from build123d import *

# Parameters (mm, degrees)
SKETCH_W        = 13.8
SKETCH_H        = 7.2
SKETCH_R        = 2.6
SKETCH_R_2      = 1.7
PAD_DEPTH       = 3
SKETCH001_R     = 2.6
SKETCH001_R_2   = 1.7
PAD001_DEPTH    = 20
CHAMFER_SIZE    = 0.5
CHAMFER001_SIZE = 0.5
CHAMFER002_SIZE = 0.5
SKETCH002_R     = 2
SKETCH002_R_2   = 1.5
PAD002_DEPTH    = 1
CHAMFER003_SIZE = 0.15
CHAMFER004_SIZE = 0.5


with BuildPart() as part:
    # Sketch → Pad (new body)
    with BuildSketch(Plane.XY):
        with Locations((3.3, 0)):
            Rectangle(SKETCH_W, SKETCH_H)
        Circle(SKETCH_R, mode=Mode.SUBTRACT)
        with Locations((7.5, 0)):
            Circle(SKETCH_R_2, mode=Mode.SUBTRACT)
    extrude(amount=PAD_DEPTH)

    # Sketch001 → Pad001 (new body)
    with BuildSketch(Plane.XY.offset(3)):
        Polygon((5.7, -2.7), (9.3, -2.7), (10.2, -1.8), (10.2, 1.8), (9.3, 2.7), (5.7, 2.7), (4.8, 3.6), (-3.6, 3.6), (-3.6, -3.6), (4.8, -3.6), align=None)
        Circle(SKETCH001_R, mode=Mode.SUBTRACT)
        with Locations((7.5, 0)):
            Circle(SKETCH001_R_2, mode=Mode.SUBTRACT)
    extrude(amount=PAD001_DEPTH)

    # Chamfer
    chamfer_edges = [part.edges().sort_by_distance(p)[0] for p in [
        (5.25, -3.15, 3),
        (7.5, -2.7, 3),
        (9.75, -2.25, 3),
        (9.75, 2.25, 3),
        (7.5, 2.7, 3),
        (5.25, 3.15, 3),
    ]]
    chamfer(chamfer_edges, length=CHAMFER_SIZE)

    # Chamfer001
    chamfer001_edges = [part.edges().sort_by_distance(p)[0] for p in [
        (0.6, -3.6, 23),
        (-3.6, 0, 23),
        (0.6, 3.6, 23),
        (5.25, 3.15, 23),
        (7.5, 2.7, 23),
        (9.75, 2.25, 23),
        (10.2, 0, 23),
        (9.75, -2.25, 23),
        (7.5, -2.7, 23),
        (5.25, -3.15, 23),
    ]]
    chamfer(chamfer001_edges, length=CHAMFER001_SIZE)

    # Chamfer002
    chamfer002_edges = [part.edges().sort_by_distance(p)[0] for p in [
        (10.2, -3.6, 1.5),
        (10.2, 3.6, 1.5),
    ]]
    chamfer(chamfer002_edges, length=CHAMFER002_SIZE)

    # Sketch002 → Pad002 (new body)
    with BuildSketch(Plane.XY.offset(23)):
        with Locations((7.5, 0)):
            Circle(SKETCH002_R)
        with Locations((7.5, 0)):
            Circle(SKETCH002_R_2, mode=Mode.SUBTRACT)
    extrude(amount=-PAD002_DEPTH)

    # Chamfer003
    chamfer003_edges = [part.edges().sort_by_distance(p)[0] for p in [
        (5.8, 0, 22),
    ]]
    chamfer(chamfer003_edges, length=CHAMFER003_SIZE)

    # Chamfer004
    chamfer004_edges = [part.edges().sort_by_distance(p)[0] for p in [
        (-3.6, 3.6, 12.75),
        (-3.6, 3.6, 1.5),
        (-3.6, -3.6, 1.5),
        (-3.6, -3.6, 12.75),
    ]]
    chamfer(chamfer004_edges, length=CHAMFER004_SIZE)


solid = part.part
The model under review builds one solid part; all positions refer to its coordinate system, in mm. A direction names the side the tool comes from. Coordinates: 2 decimals unless noted, no trailing zeros. Write each loop counter-clockwise with the first axis right and the second up, starting at its lowest first coordinate (ties: lowest second). Pieces come first, ordered by that corner, then holes. Notation, with made-up numbers: (77.25, 12) - (88.25, 12) arc R29 cw to (88.25, 42) - close; hole circle Ø10 at (39.25, 54.5). An arc over 180 degrees is marked (long way). Answer as a JSON object with one key per item and string values. Group by question number.
1. Add section D-D (x = 0). Give the boundary of the cut face in (y, z).
2. To check wall thickness, follow probe 1 along X at (y, z) = (0.5, 21.5); probe 2 along Y at (x, z) = (7.5, 16.5); probe 3 along X at (y, z) = (1.5, 17.5). State the ranges of each line that lie inside material, in increasing order.
3. Mouldability with a two-part tool opening along X and no side actions: class faces 4 (the face through (-0.338, 2.578, 11.339)), 5 (the face through (5.3, 3.1, 12.9)), 6 (the face through (1, 3.6, 11)) as pulls with the +X half, pulls with the -X half, needs draft (parallel to the pull), parting line crosses it, or undercut.
4. Add section A-A (x = 7.5). Give the boundary of the cut face in (y, z), plus the area to 3 significant figures.
5. Clearance check with flat-ended pins moving along their axes: pin 1 Ø1.2 at (x, y) = (8, 3) entering from +Z; pin 2 Ø1.8 at (x, z) = (7, 16.5) entering from -Y; pin 3 Ø0.5 at (x, y) = (7.5, -3) entering from +Z. State where each tip first meets the part, or that it passes through.
6. Add section B-B (z = 14.25). Give the boundary of the cut face in (x, y).
7. Add section C-C (y = 0). Give the boundary of the cut face in (x, z), plus the area to 3 significant figures.
8. Machinability: for faces 1 (the face through (6.15, -1.03, 10.77)), 2 (the face through (10, 2, 13)), 3 (the face through (10, -2, 13)), which of the approach directions +Z, -Z, +X, -X, +Y, -Y give a long, thin tool a straight path to every point of the face, cutting with its end or side? Answer none if there is none.
Findings:
{
 "1": {"outline": "(-3.6, 0) - (-2.6, 0) - (-2.6, 23) - (-3.1, 23) - (-3.6, 22.5) - close; (2.6, 0) - (3.6, 0) - (3.6, 22.5) - (3.1, 23) - (2.6, 23) - close"},
 "2": {"probe 1": "-3.6 to -2.55, 2.55 to 5.88, 9.12 to 10.2", "probe 2": "-2.7 to -1.7, 1.7 to 2.7", "probe 3": "-3.6 to -2.12, 2.12 to 6.7, 8.3 to 10.2"},
 "3": {"face 4": "undercut", "face 5": "pulls with the +X half", "face 6": "needs draft"},
 "4": {"outline": "(-3.6, 0) - (-1.7, 0) - (-1.7, 21.85) - (-1.55, 22) - (-1.5, 22) - (-1.5, 23) - (-2.2, 23) - (-2.7, 22.5) - (-2.7, 3.5) - (-3.2, 3) - (-3.6, 3) - close; (1.5, 22) - (1.55, 22) - (1.7, 21.85) - (1.7, 0) - (3.6, 0) - (3.6, 3) - (3.2, 3) - (2.7, 3.5) - (2.7, 22.5) - (2.2, 23) - (1.5, 23) - close", "area": "51.8 mm²"},
 "5": {"pin 1": "z = 22.8", "pin 2": "y = -2.7", "pin 3": "z = 3.45"},
 "6": {"outline": "(-3.6, -3.1) - (-3.1, -3.6) - (4.8, -3.6) - (5.7, -2.7) - (9.3, -2.7) - (10.2, -1.8) - (10.2, 1.8) - (9.3, 2.7) - (5.7, 2.7) - (4.8, 3.6) - (-3.1, 3.6) - (-3.6, 3.1) - close; hole circle Ø5.2 at (0, 0); hole circle Ø3.4 at (7.5, 0)"},
 "7": {"outline": "(-3.6, 0) - (-2.6, 0) - (-2.6, 23) - (-3.1, 23) - (-3.6, 22.5) - close; (2.6, 0) - (5.8, 0) - (5.8, 21.85) - (5.95, 22) - (6, 22) - (6, 23) - (2.6, 23) - close; (9, 22) - (9.05, 22) - (9.2, 21.85) - (9.2, 0) - (10.2, 0) - (10.2, 22.5) - (9.7, 23) - (9, 23) - close", "area": "120 mm²"},
 "8": {"face 1": "-Z", "face 2": "+Z, +X, +Y", "face 3": "+Z, +X, -Y"}
}
